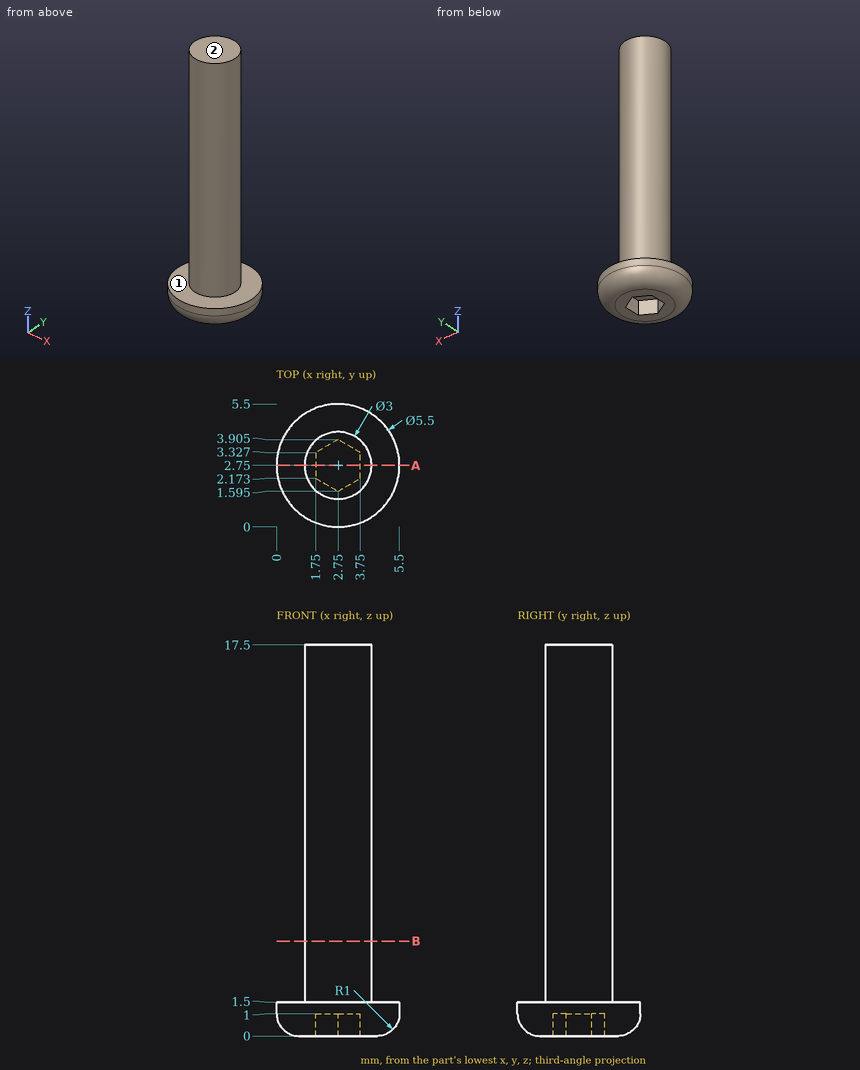
Source: three-view drawing plus pictorial views. Frame: mm from the lowest corner of the part. A direction names the side the tool comes from. Give positions to 0.01 mm unless a question says otherwise; leave off trailing zeros. Order: outer loops, then holes, each group sorted by start corner. A loop starts at its lowest first (then second) coordinate and runs counter-clockwise, first axis right, second up. Notation, with made-up numbers: (-23, 30.25) -> (-1, 30.25) arc R5 cw to (-1, 35.25) -> close; hole circle Ø7 at (86, 88). An arc over 180 degrees is marked (long way). Use a Markdown table: item, result.
Q1. Material intervals for line 1 (Z direction, x = 3.4, y = 2.8); line 2 (Z direction, x = 1.15, y = 2.35); line 3 (Y direction, x = 2.75, z = 3), sorted ascending. Write a range as [from, to].
A:
| item | result |
|---|---|
| line 1 | [1, 17.5] |
| line 2 | [0, 1.5] |
| line 3 | [1.25, 4.25] |
Q2. First-contact query: P1, Ø0.5, axis at y = 2.5, z = 0.5, coming from the +X side; P2, Ø0.8, axis at y = 2.5, z = 0.5, coming from the -X side; P3, Ø0.6, axis at x = 3, y = 3, coming from the -Z side. Flat tips, straight axial feed; report the tip coordinate or a pass-through.
A:
| item | result |
|---|---|
| P1 | x = 5.46 |
| P2 | x = 0.01 |
| P3 | z = 1 |
Q3. Section B-B (z = 4.25). Return the cut outline in (x, y).
A:
| item | result |
|---|---|
| outline | circle Ø3 at (2.75, 2.75) |
Q4. Access query for the marked faces 1 and 2. Directions: +Z, -Z, +X, -X, +Y, -Y. A direction counts if a zero-diameter tool reaches every point of the face in a straight line with its end or side. Return the directions, or none.
A:
| item | result |
|---|---|
| face 1 | +Z |
| face 2 | +Z, +X, -X, +Y, -Y |
Q5. Section A-A (y = 2.75). Return the cut outline in (x, z).
A:
| item | result |
|---|---|
| outline | (0, 1) arc R1 ccw to (1, 0) -> (1.75, 0) -> (1.75, 1) -> (3.75, 1) -> (3.75, 0) -> (4.5, 0) arc R1 ccw to (5.5, 1) -> (5.5, 1.5) -> (4.25, 1.5) -> (4.25, 17.5) -> (1.25, 17.5) -> (1.25, 1.5) -> (0, 1.5) -> close |
